Could you check a few things on this model? Use its own coordinates, in mm. Face numbers are marked on the shaded views. Coordinates: 2 decimals unless noted, no trailing zeros. Loops run counter-clockwise (first coordinate to the right, second up) from the corner with the lowest first, then second, coordinate; pieces in that order, holes last.
from build123d import *

# Parameters (mm, degrees)
SKETCH1_R               = 16.7005
SKETCH1_R_2             = 13.0683
BOSS_EXTRUDE1_DEPTH     = 254
CUT_EXTRUDE2_DEPTH      = 256.095694594
CUT_EXTRUDE2_DEPTH_BACK = 256.095694594
SKETCH3_R               = 3.2639
SKETCH4_R               = 3.2639
CUT_EXTRUDE3_DEPTH      = 256.095694707
CUT_EXTRUDE4_START      = -79.375
SKETCH5_R               = 16.7005
CUT_EXTRUDE4_DEPTH      = 79.375
SKETCH7_R               = 16.7005
CUT_EXTRUDE6_DEPTH      = 3.175


with BuildPart() as part:
    # Sketch1 → Boss-Extrude1 (new body)
    with BuildSketch(Plane(origin=(0, 0, 0), x_dir=(0, 0, -1), z_dir=(1, 0, 0))):
        Circle(SKETCH1_R)
        Circle(SKETCH1_R_2, mode=Mode.SUBTRACT)
    extrude(amount=BOSS_EXTRUDE1_DEPTH)

    # Sketch3 → Cut-Extrude2 (cut, two sides: drawn at the far end of the back side and taken through both)
    with BuildSketch(Plane(origin=(0, 0, 0), x_dir=(1, 0, 0), z_dir=(0, 1, 0)).offset(-CUT_EXTRUDE2_DEPTH_BACK)):
        with Locations(Location((127, 0, 0), (0, 0, 270))):
            Circle(SKETCH3_R)
    extrude(amount=CUT_EXTRUDE2_DEPTH + CUT_EXTRUDE2_DEPTH_BACK, mode=Mode.SUBTRACT)

    # Sketch4 → Cut-Extrude3 (cut, symmetric)
    with BuildSketch(Plane(origin=(0, 0, 0), x_dir=(-1, 0, 0), z_dir=(0, 0.819152044288991, -0.5735764363510473))):
        with Locations(Location((-203.2, 0, 0), (0, 0, 90))):
            Circle(SKETCH4_R)
        with Locations(Location((-50.8, 0, 0), (0, 0, 90))):
            Circle(SKETCH4_R)
    cut_extrude3 = extrude(amount=CUT_EXTRUDE3_DEPTH, both=True, mode=Mode.SUBTRACT)

    # Sketch5 → Cut-Extrude4 (cut)
    with BuildSketch(Plane(origin=(254, 0, 0), x_dir=(0, 0, -1), z_dir=(1, 0, 0)).offset(CUT_EXTRUDE4_START)):
        Circle(SKETCH5_R)
    extrude(amount=CUT_EXTRUDE4_DEPTH, mode=Mode.SUBTRACT)

    # Mirror1: Cut-Extrude3 across plane
    add(cut_extrude3.mirror(Plane.XY), mode=Mode.SUBTRACT)

    # Sketch7 → Cut-Extrude6 (cut)
    with BuildSketch(Plane.ZY):
        Circle(SKETCH7_R)
    extrude(amount=-CUT_EXTRUDE6_DEPTH, mode=Mode.SUBTRACT)


solid = part.part
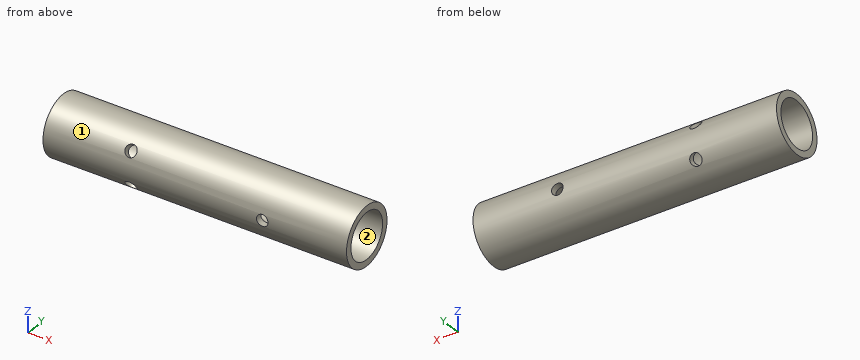
(1) We'd pull the mould along Y, two halves only. Please class the marked faces 1 and 2: +Y half, -Y half, draft (parallel to the pull), parting line (faces both ways), or undercut.
Answers:
face 1: parting line
face 2: undercut
(2) Imagine slicing it at C-C, the plane x = 127. Write out the boundary of the cut face in (y, z), and give its area (3 significant figures).
Answers:
outline: (-16.38, -3.26) arc R16.7 ccw to (16.38, -3.26) - (12.65, -3.26) arc R13.07 cw to (-12.65, -3.26) - close; (-16.38, 3.26) - (-12.65, 3.26) arc R13.07 cw to (12.65, 3.26) - (16.38, 3.26) arc R16.7 ccw to start
area: 292 mm2
(3) For pin 1 (4 mm diameter, centred on x = 127, z = 0, fed in from +Y); pin 2 (1.5 mm diameter, centred on x = 67.5, y = -5.5, fed in from +Z); pin 3 (6 mm diameter, centred on x = 60, y = -6, fed in from +Z); pin 4 (6 mm diameter, centred on x = 103.5, z = -12.5, fed in from +Y), each with a flat end and sliding along its axis, tell me the tip position at first contact or that it passes through.
Answers:
pin 1: passes through
pin 2: stops at z = 16.01
pin 3: stops at z = 16.43
pin 4: stops at y = 13.74
(4) Imagine slicing it at D-D, the plane x = 89. Write out the boundary of the cut face in (y, z).
Answers:
outline: circle Ø33.4 at (0, 0); hole circle Ø26.14 at (0, 0)
(5) Imagine slicing it at A-A, the plane y = 0. Write out the boundary of the cut face in (x, z) (1 decimal), and give its area (3 significant figures).
Answers:
outline: (3.2, -16.7) - (174.6, -16.7) - (174.6, -13.1) - (3.2, -13.1) - close; (3.2, 13.1) - (174.6, 13.1) - (174.6, 16.7) - (3.2, 16.7) - close
area: 1,250 mm2
(6) Imagine slicing it at B-B, the plane z = 0. Write out the boundary of the cut face in (x, y) (1 decimal), and give its area (3 significant figures).
Answers:
outline: (3.2, -16.7) - (123.7, -16.7) - (123.7, -13.1) - (3.2, -13.1) - close; (3.2, 13.1) - (123.7, 13.1) - (123.7, 16.7) - (3.2, 16.7) - close; (130.3, -16.7) - (174.6, -16.7) - (174.6, -13.1) - (130.3, -13.1) - close; (130.3, 13.1) - (174.6, 13.1) - (174.6, 16.7) - (130.3, 16.7) - close
area: 1,200 mm2
(7) I need wall thicknesses on probe 1 along Y at (x, z) = (130.5, 0); probe 2 along X at (y, z) = (15.2, 0) (3 decimals); probe 3 along X at (y, z) = (-13, -2.5) (3 decimals). Which ranges of each line are inside material? Lowest first, please.
Answers:
probe 1: y = -16.7 to -13.07, 13.07 to 16.7
probe 2: x = 3.175 to 123.736, 130.264 to 174.625
probe 3: x = 3.175 to 124.902, 129.098 to 174.625
